Autodesk Inventor part; units mm, degrees
ref_plane "YZ Plane" through (0, 0, 0) normal (1, 0, 0) x (0, 1, 0)
ref_plane "XZ Plane" through (0, 0, 0) normal (0, 1, 0) x (-1, 0, 0)
ref_plane "XY Plane" through (0, 0, 0) normal (0, 0, 1) x (1, 0, 0)
sketch "Sketch1" plane through (0, 0, 0) normal (0, 1, 0) x (-1, 0, 0)
  line L0 (0, 0) -> (350, 0)
  line L1 (350, 0) -> (350, -100)
  line L2 (350, -100) -> (0, -100)
  line L3 (0, -100) -> (0, 0)
  dimension "d0" = 350
  dimension "d1" = 100
extrude "Extrusion1" add sketch "Sketch1" along normal blind 6.35
sketch "Sketch2" plane through (0, 6.35, 0) normal (0, 1, 0) x (1, 0, 0)
  line L0 (0, 100) -> (-350, 100)
  line L1 (-192.5, 100) -> (-157.5, 100)
  line L2 (-157.5, 100) -> (-157.5, 60)
  line L3 (-157.5, 60) -> (-192.5, 60)
  line L4 (-192.5, 60) -> (-192.5, 100)
  line L5 (0, 0) -> (0, 100)
  dimension "d10" = 35
  dimension "d11" = 40
  dimension "d12" = 157.5
extrude "Extrusion2" add sketch "Sketch2" along normal blind 62
sketch "Sketch3" plane through (0, 68.35, 0) normal (0, 1, 0) x (1, 0, 0)
  circle A0 centre (-175, 94) radius 2.125
  line L0 (-157.5, 100) -> (-192.5, 100)
  circle A1 centre (-169, 94) radius 2.125
  circle A2 centre (-181, 94) radius 2.125
  point P0 (0, 0)
  dimension "d15" = 4.25
  dimension "d16" = 6
  dimension "d17" = 4.25
  dimension "d18" = 6
  dimension "d19" = 4.25
  dimension "d20" = 6
hole "Hole1" at (-181, 68.35, -94) at (-175, 68.35, -94) at (-169, 68.35, -94) direction (0, -1, 0) diameter 4.25 depth 8 tip angle 118
sketch "Sketch4" plane through (-192.5, 6.35, -100) normal (-1, 0, 0) x (0, 0, 1)
  point P0 (100, -6.35)
sketch "Sketch5" plane through (-192.5, 6.35, -100) normal (-1, 0, 0) x (0, 0, 1)
  line L0 (0, 0) -> (0, 62)
  line L1 (0, 42) -> (40, 42)
  line L2 (40, 0) -> (40, 62)
  line L3 (0, 62) -> (40, 62)
  circle A0 centre (6, 48) radius 1.5
  circle A1 centre (34, 48) radius 1.5
  point P0 (100, -6.35)
  dimension "d28" = 20
  dimension "d29" = 3
  dimension "d30" = 3
  dimension "d31" = 6
  dimension "d32" = 6
  dimension "d33" = 6
  dimension "d34" = 6
hole "Hole2" at (-192.5, 54.35, -66) at (-192.5, 54.35, -94) direction (1, 0, 0) diameter 3 depth 2 tip angle 118
sketch "Sketch6" plane through (-192.5, 6.35, -60) normal (0, 0, 1) x (1, 0, 0)
  line L0 (0, 42) -> (35, 42)
  line L1 (0, 62) -> (35, 62)
  circle A0 centre (6, 48) radius 1.5
  line L2 (0, 0) -> (0, 62)
  circle A1 centre (29, 48) radius 1.5
  line L3 (35, 0) -> (35, 62)
  point P0 (192.5, -6.35)
  dimension "d42" = 20
  dimension "d43" = 3
  dimension "d44" = 6
  dimension "d45" = 6
  dimension "d46" = 3
  dimension "d47" = 6
  dimension "d48" = 6
hole "Hole3" at (-186.5, 54.35, -60) at (-163.5, 54.35, -60) direction (0, 0, -1) diameter 3 depth 2 tip angle 118
sketch "Sketch7" plane through (-157.5, 6.35, -60) normal (1, 0, 0) x (0, 0, -1)
  circle A0 centre (6, 48) radius 1.5
  circle A1 centre (6, 48) radius 1.5
  circle A2 centre (34, 48) radius 1.5
  circle A3 centre (34, 48) radius 1.5
  point P0 (-60, -6.35)
  dimension "d56" = 3
  dimension "d57" = 3
hole "Hole4" at (-157.5, 54.35, -66) at (-157.5, 54.35, -94) direction (-1, 0, 0) diameter 3 depth 2 tip angle 118
sketch "Sketch8" plane through (0, 0, 0) normal (0, -1, 0) x (1, 0, 0)
  line L0 (-350, -100) -> (0, -100)
  line L1 (-350, -100) -> (-330, -100)
  line L2 (-330, 0) -> (-330, 255)
  line L3 (-330, 325) -> (-350, 325)
  line L4 (-350, 325) -> (-350, 0)
  line L5 (-350, 325) -> (0, 325)
  line L6 (0, 0) -> (0, -100)
  line L7 (0, 325) -> (0, 0)
  line L8 (0, -100) -> (-20, -100)
  line L9 (0, -100) -> (-157.5, -100)
  line L10 (-20, 0) -> (-20, 255)
  line L11 (-20, 325) -> (50, 325) construction
  line L12 (-20, 255) -> (-330, 255)
  line L13 (-350, 0) -> (0, 0)
  line L14 (-350, 0) -> (-330, 0)
  line L15 (-20, 0) -> (0, 0)
  dimension "d65" = 20
  dimension "d66" = 425
extrude "Extrusion3" add sketch "Sketch8" against normal blind 7.5 contours L13 L4 L3 L5 L7 L10 L12 L2
sketch "Sketch9" plane through (0, 7.5, 0) normal (0, 1, 0) x (1, 0, 0)
  line L0 (-20, -255) -> (-330, -255)
  line L1 (-175, -255) -> (-175, -325)
  line L2 (-350, -325) -> (0, -325)
  line L3 (-175, -290) -> (-168, -290)
  line L4 (0, 100) -> (0, -325)
  line L5 (-168, -290) -> (-134.9357, -290)
  circle A0 centre (-175, -290) radius 5
  circle A1 centre (-105, -290) radius 5
  circle A2 centre (-245, -290) radius 5
  point P0 (0, 0)
  dimension "d73" = 7
  dimension "d74" = 10
  dimension "d75" = 10
  dimension "d76" = 10
  dimension "d77" = 70
  dimension "d78" = 70
hole "Hole5" at (-105, 7.5, 290) at (-175, 7.5, 290) at (-245, 7.5, 290) direction (0, -1, 0) diameter 10 depth 8 tip angle 118
properties part number "Base" material "Wood (Birch)"
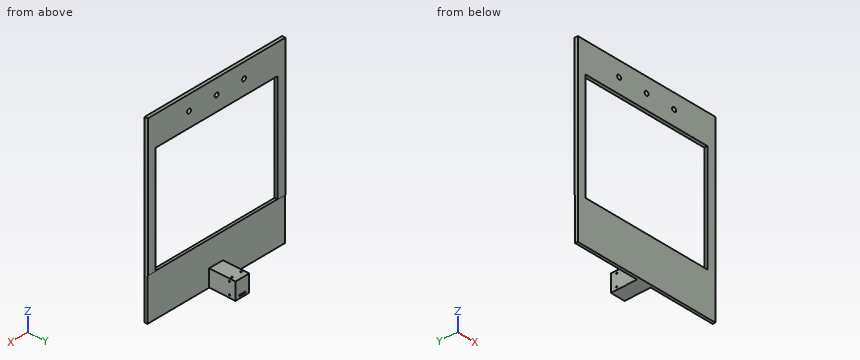
The listing builds one solid part. Answer for the finished solid, in the listing's coordinates (mm). Coordinates: 2 decimals unless noted, no trailing zeros. Write each loop counter-clockwise with the first axis right and the second up, starting at its lowest first coordinate (ties: lowest second). Pieces come first, ordered by that corner, then holes.
Q1. Given P1, Ø6, axis at x = -69, z = 256.5, coming from the -Y side; P2, Ø2.5, axis at y = 54.35, z = -94, coming from the -X side; P3, Ø12, axis at y = 42, z = -84, coming from the -X side; P4, Ø5, axis at x = -163.5, y = 54.35, coming from the +Z side, each flat-ended and moving along its own axis, determine where each tip first touches the part or whether it passes through.
Returned:
P1: stops at y = 0
P2: stops at x = -190.35
P3: stops at x = -192.5
P4: stops at z = -60
Q2. Find the intervals of material crossed by line 1 along Z through (x, y) = (-191.8, 54.35); line 2 along X through (y, z) = (6, 290); line 3 along X through (y, z) = (62, -94) (3 decimals), in increasing order.
Returned:
line 1: z = -100 to -95.5, -92.5 to -67.5, -64.5 to -60
line 2: x = -350 to -250, -240 to -180, -170 to -110, -100 to 0
line 3: x = -192.5 to -183.125, -178.875 to -177.125, -172.875 to -171.125, -166.875 to -157.5
Q3. Section C-C, the plane z = 290 is taken. Write down the section's boundary in (x, y).
Returned:
outline: (-350, 0) - (-250, 0) - (-250, 7.5) - (-350, 7.5) - close; (-240, 0) - (-180, 0) - (-180, 7.5) - (-240, 7.5) - close; (-170, 0) - (-110, 0) - (-110, 7.5) - (-170, 7.5) - close; (-100, 0) - (0, 0) - (0, 7.5) - (-100, 7.5) - close
Q4. Section A-A, the plane x = -290.5 is taken. Write down the section's boundary in (y, z), then the cut area to 3 significant figures.
Returned:
outline: (0, -100) - (6.35, -100) - (6.35, 0) - (0, 0) - close; (0, 255) - (7.5, 255) - (7.5, 325) - (0, 325) - close
area: 1,160 mm2
Q5. Section D-D, the plane z = -72.5 is taken. Write down the section's boundary in (x, y).
Returned:
outline: (-350, 0) - (0, 0) - (0, 6.35) - (-157.5, 6.35) - (-157.5, 68.35) - (-192.5, 68.35) - (-192.5, 6.35) - (-350, 6.35) - close
Q6. Section B-B, the plane z = 76 is taken. Write down the section's boundary in (x, y).
Returned:
outline: (-350, 0) - (-330, 0) - (-330, 7.5) - (-350, 7.5) - close; (-20, 0) - (0, 0) - (0, 7.5) - (-20, 7.5) - close
